Can you work these out from the model? Positions are in its coordinate system, mm. Face numbers are marked on the shaded views. A direction names the side the tool comes from. Round coordinates to 2 decimals unless told otherwise and drop trailing zeros. Order: outer loops, then holes, each group sorted by start corner. A loop starts at its lowest first (then second) coordinate and runs counter-clockwise, first axis right, second up. Notation, with made-up numbers: M -26,-36.75 L -4,-36.75 A21 cw -4,-21.75 Z; hole C -3.5,-3.5 d4. An arc over 180 degrees is marked long. Answer as a JSON object with one key per item and string values. Group by question number.
```python
from build123d import *

# Parameters (mm, degrees)
SKETCH1_R               = 6
SKETCH1_R_2             = 2.5
BOSS_EXTRUDE1_DEPTH     = 9
SKETCH2_R               = 5
SKETCH2_R_2             = 1.475
BOSS_EXTRUDE2_DEPTH     = 6
BOSS_EXTRUDE3_DEPTH     = 6
CUT_EXTRUDE2_DEPTH      = 17.155494421
CUT_EXTRUDE2_DEPTH_BACK = 17.155494421
SKETCH5_R               = 1.475
SKETCH5_W               = 8.5
SKETCH5_H               = 12


with BuildPart() as part:
    # Sketch1 → Boss-Extrude1 (new, symmetric)
    with BuildSketch(Plane.XY):
        with Locations((-6, 0)):
            Circle(SKETCH1_R)
        with Locations((-6, 0)):
            Circle(SKETCH1_R_2, mode=Mode.SUBTRACT)
    extrude(amount=BOSS_EXTRUDE1_DEPTH, both=True)

    # Sketch2 → Boss-Extrude2 (add, symmetric)
    with BuildSketch(Plane(origin=(0, 0, 0), x_dir=(1, 0, 0), z_dir=(0, 1, 0))):
        with Locations(Location((0, 0, 0), (0, 0, 270))):
            Circle(SKETCH2_R)
        with Locations(Location((0, 0, 0), (0, 0, 270))):
            Circle(SKETCH2_R_2, mode=Mode.SUBTRACT)
    extrude(amount=BOSS_EXTRUDE2_DEPTH, both=True)

    # Sketch4 → Boss-Extrude3 (add, symmetric)
    with BuildSketch(Plane(origin=(0, 0, 0), x_dir=(1, 0, 0), z_dir=(0, 1, 0))):
        with BuildLine():
            Line((-6, 9), (-6, -9))
            Line((-6, -9), (0, -9))
            Line((0, -9), (4.157397096, -2.777777778))
            ThreePointArc((4.157397096, -2.777777778), (5, 0), (4.157397096, 2.777777778))
            Line((4.157397096, 2.777777778), (0, 9))
            Line((0, 9), (-6, 9))
        make_face()
    extrude(amount=BOSS_EXTRUDE3_DEPTH, both=True)

    # Sketch3 → Cut-Revolve1 (revolve, cut)
    with BuildSketch(Plane(origin=(0, 0, 0), x_dir=(1, 0, 0), z_dir=(0, 1, 0)), mode=Mode.PRIVATE) as cut_revolve1_sk:
        Polygon((-3.5, 8), (-3.5, 9), (-6, 9), (-6, -9), (-3.5, -9), (-3.5, -8), (-3, -8), (-3, -6), (-1.5, -6), (-1.5, 6), (-3, 6), (-3, 8), align=None)
    revolve(cut_revolve1_sk.sketch.rotate(Axis((-6, 0, -12.234149704), (0, 0, 1)), 180), axis=Axis((-6, 0, -12.234149704), (0, 0, 1)), mode=Mode.SUBTRACT)

    # Sketch5 → Cut-Extrude2 (cut, two sides: drawn at the far end of the back side and taken through both)
    with BuildSketch(Plane(origin=(0, 0, 0), x_dir=(1, 0, 0), z_dir=(0, 1, 0)).offset(-CUT_EXTRUDE2_DEPTH_BACK)):
        with Locations(Location((0, 0, 0), (0, 0, 270))):
            Circle(SKETCH5_R)
        with Locations((-7.75, 0)):
            Rectangle(SKETCH5_W, SKETCH5_H)
    extrude(amount=CUT_EXTRUDE2_DEPTH + CUT_EXTRUDE2_DEPTH_BACK, mode=Mode.SUBTRACT)


solid = part.part
```
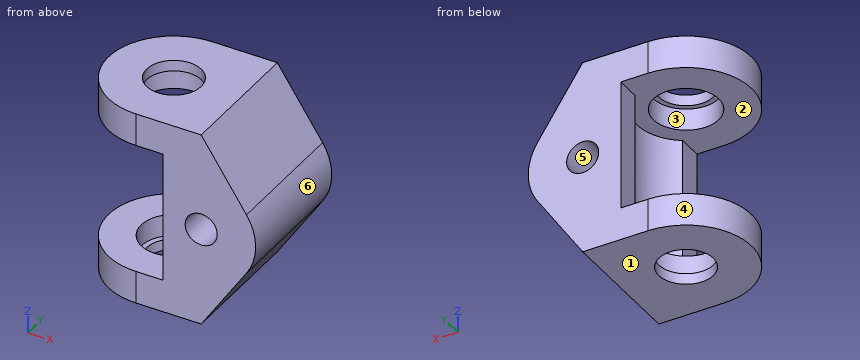
1) For pin 1 (1.8 mm diameter, centred on x = -5, y = 0.5, fed in from +Z); pin 2 (2 mm diameter, centred on x = 3, y = 0.5, fed in from +Z); pin 3 (1.1 mm diameter, centred on y = -5, z = -1, fed in from -X), each with a flat end and sliding along its axis, tell me the tip position at first contact or that it passes through.
2) I need wall thicknesses on line 1 along Z through (x, y) = (-9, -0.75); line 2 along Y through (x, z) = (-6, -7.5); line 3 along Y through (x, z) = (-6, -8.2). Which ranges of each line are inside material? Lowest first, please.
3) If we section it at A-A on y = 0: Write out the boundary of the cut face in (x, z) (3 decimals).
4) If we section it at B-B on z = 0: Write out the boundary of the cut face in (x, y) (3 decimals), plus the area to 3 significant figures.
5) If we section it at C-C on x = -2.75: Write out the boundary of the cut face in (y, z).
6) Which directions (+Z, -Z, +X, -X, +Y, -Y) give clear straight access to the entire face, cutting with the end or side of a thin tool? Please do the marked faces 1, 2 and 3.
7) We'd pull the mould along X, two halves only. Please class the marked faces 4, 5 and 6: +X half, -X half, draft (parallel to the pull), parting line (faces both ways), or undercut.
8) If we section it at D-D on y = 5: Write out the boundary of the cut face in (x, z) (3 decimals), plus the area to 3 significant figures.
Findings:
{
 "1": {"pin 1": "passes through", "pin 2": "stops at z = 6.01", "pin 3": "stops at x = -3.5"},
 "2": {"line 1": "z = -9 to -6, 6 to 9", "line 2": "y = -6 to -3, 3 to 6", "line 3": "y = -6 to -2.5, 2.5 to 6"},
 "3": {"outline": "M -12,-9 L -8.5,-9 L -8.5,-8 L -9,-8 L -9,-6 L -12,-6 Z; M -12,6 L -9,6 L -9,8 L -8.5,8 L -8.5,9 L -12,9 Z; M -3.5,-9 L 0,-9 L 4.157,-2.778 A5 ccw 4.157,2.778 L 0,9 L -3.5,9 L -3.5,8 L -3,8 L -3,6 L -1.5,6 L -1.5,-6 L -3,-6 L -3,-8 L -3.5,-8 Z; hole C 0,0 d2.95"},
 "4": {"outline": "M -3.5,-6 L -1.475,-6 L -1.475,6 L -3.5,6 L -3.5,3.742 A4.5 cw -3.5,-3.742 Z; M 1.475,-6 L 5,-6 L 5,6 L 1.475,6 Z", "area": "56.1 mm^2"},
 "5": {"outline": "M -6,-9 L 6,-9 L 6,9 L -6,9 Z; hole M -3.11,-6 L 3.11,-6 L 3.11,6 L -3.11,6 Z"},
 "6": {"face 1": "-Z, +X, -X, +Y, -Y", "face 2": "-X", "face 3": "none"},
 "7": {"face 4": "-X half", "face 5": "undercut", "face 6": "+X half"},
 "8": {"outline": "M -9.317,-9 L 0,-9 L 4.157,-2.778 A5 ccw 4.157,2.778 L 0,9 L -9.317,9 L -9.317,6 L -3.5,6 L -3.5,-6 L -9.317,-6 Z; hole C 0,0 d2.95", "area": "143 mm^2"}
}
